Study the drawing (mm; zero at the part's minimum x, y, z) and answer. A direction names the side the tool comes from. Round coordinates to 2 decimals unless told otherwise and drop trailing zeros. Order: outer loops, then holes, each group sorted by start corner. A loop starts at its lowest first (then second) coordinate and runs counter-clockwise, first axis right, second up. Notation, with made-up numbers: (67.25, 3) -> (106.25, 3) arc R23 cw to (106.25, 16) -> close; hole circle Ø3 at (-7, 16). An arc over 180 degrees is marked (long way). Answer in a Markdown table with one row per item. Add a question column.
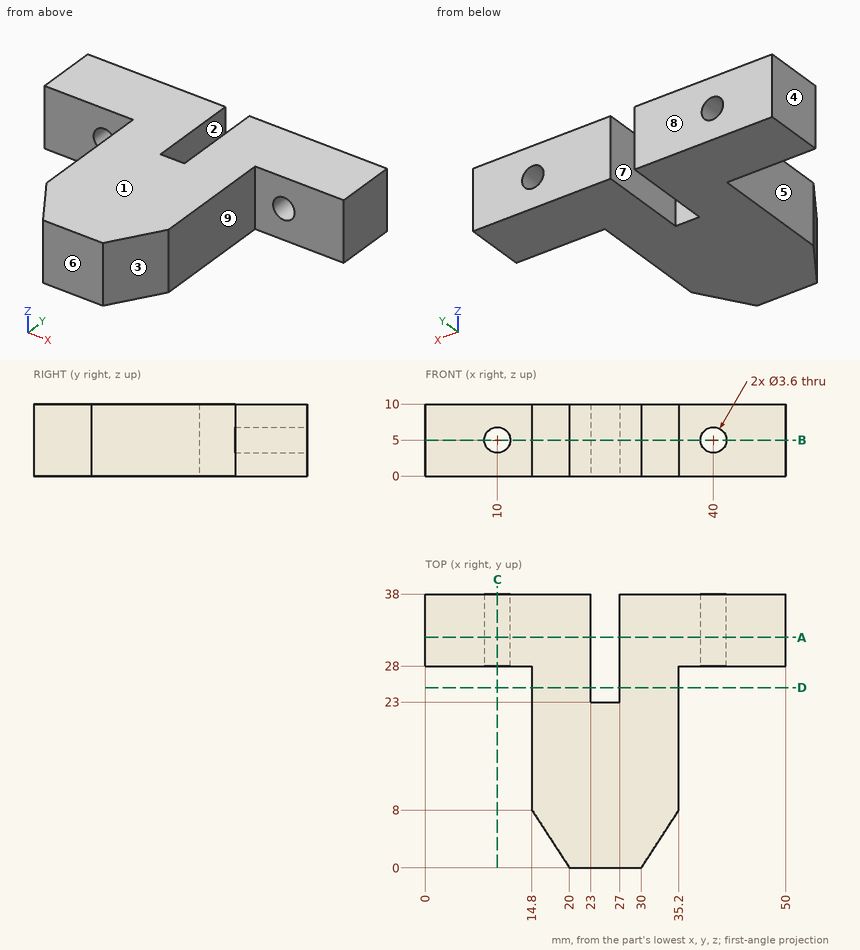
Item 1: Find the intervals of material crossed by probe 1 along X at (y, z) = (24, 4.5); probe 2 along X at (y, z) = (31.5, 1.75); probe 3 along Z at (x, y) = (10, 31), in increasing order. Write a range as [from, to].
Item 2: Flat-ended cylindrical pins translate along their axes: P1, Ø3, axis at y = 18.5, z = 4, coming from the +X side; P2, Ø2, axis at y = 11, z = 5, coming from the -X side; P3, Ø3, axis at x = 4.5, z = 5, coming from the -Y side. Find the tip coordinate at first contact, or state that the pin passes through.
Item 3: The part is cut by section D-D, the plane y = 25. Give the vertices of the cut face in (x, z).
Item 4: A tool of negligible diameter and unlimited length cuts with its end or side. For the marked faces 5, 6, 7, 8 and 9, from which of +Z, -Z, +X, -X, +Y, -Y can it reach the whole face along a straight path? Write none if from no direction.
Item 5: The part is cut by section C-C, the plane x = 10. Give the vertices of the cut face in (y, z).
Item 6: For a pull along X with two mould halves and no side action, classify the marked faces 1, 2, 3 and 4 as released by +X, released by -X, zero draft, split by the parting line, or undercut.
Item 7: The part is cut by section B-B, the plane z = 5. Give the vertices of the cut face in (x, y).
Item 8: The part is cut by section A-A, the plane y = 32. Give the vertices of the cut face in (x, z), and give its area (3 significant figures).
Resolved:
| question | item | result |
|---|---|---|
| 1 | probe 1 | [14.8, 23], [27, 35.2] |
| 1 | probe 2 | [0, 23], [27, 50] |
| 1 | probe 3 | [0, 3.2], [6.8, 10] |
| 2 | P1 | x = 35.2 |
| 2 | P2 | x = 14.8 |
| 2 | P3 | y = 28 |
| 3 | outline | (14.8, 0) -> (23, 0) -> (23, 10) -> (14.8, 10) -> close; (27, 0) -> (35.2, 0) -> (35.2, 10) -> (27, 10) -> close |
| 4 | face 5 | +Z, -Z, -X, -Y |
| 4 | face 6 | +Z, -Z, +X, -X, -Y |
| 4 | face 7 | +Z, -Z, +Y |
| 4 | face 8 | +Z, -Z, +X, -X, +Y |
| 4 | face 9 | +Z, -Z, +X, -Y |
| 5 | outline | (28, 0) -> (38, 0) -> (38, 3.2) -> (28, 3.2) -> close; (28, 6.8) -> (38, 6.8) -> (38, 10) -> (28, 10) -> close |
| 6 | face 1 | zero draft |
| 6 | face 2 | undercut |
| 6 | face 3 | released by +X |
| 6 | face 4 | released by -X |
| 7 | outline | (0, 28) -> (8.2, 28) -> (8.2, 38) -> (0, 38) -> close; (11.8, 28) -> (14.8, 28) -> (14.8, 8) -> (20, 0) -> (30, 0) -> (35.2, 8) -> (35.2, 28) -> (38.2, 28) -> (38.2, 38) -> (27, 38) -> (27, 23) -> (23, 23) -> (23, 38) -> (11.8, 38) -> close; (41.8, 28) -> (50, 28) -> (50, 38) -> (41.8, 38) -> close |
| 8 | outline | (0, 0) -> (23, 0) -> (23, 10) -> (0, 10) -> close; (27, 0) -> (50, 0) -> (50, 10) -> (27, 10) -> close; hole circle Ø3.6 at (10, 5); hole circle Ø3.6 at (40, 5) |
| 8 | area | 440 mm2 |
